```python
from build123d import *

# Parameters (mm, degrees)
F0_R     = 2.25
F0_R_2   = 6
F1_DEPTH = 2
F2_R     = 19
F2_R_2   = 6
F3_DEPTH = 4.6


with BuildPart() as f1:
    # F0 (on Top) → F1 (new body)
    with BuildSketch(Plane.XY):
        with BuildLine():
            Line((29.849623, 35), (-29.849623, 35))
            ThreePointArc((-29.849623, 35), (-32.526912, 32.526912), (-35, 29.849623))
            Line((-35, 29.849623), (-35, -29.849623))
            ThreePointArc((-35, -29.849623), (-32.526912, -32.526912), (-29.849623, -35))
            Line((-29.849623, -35), (29.849623, -35))
            ThreePointArc((29.849623, -35), (32.526912, -32.526912), (35, -29.849623))
            Line((35, -29.849623), (35, 29.849623))
            ThreePointArc((35, 29.849623), (32.526912, 32.526912), (29.849623, 35))
        make_face()
        with Locations((-27.5, -27.5)):
            Circle(F0_R, mode=Mode.SUBTRACT)
        with Locations((27.5, -27.5)):
            Circle(F0_R, mode=Mode.SUBTRACT)
        Circle(F0_R_2, mode=Mode.SUBTRACT)
        with Locations((-27.5, 27.5)):
            Circle(F0_R, mode=Mode.SUBTRACT)
        with Locations((27.5, 27.5)):
            Circle(F0_R, mode=Mode.SUBTRACT)
    extrude(amount=F1_DEPTH)

    # F2 (on face) → F3 (join)
    with BuildSketch(Plane.XY.offset(2)):
        Circle(F2_R)
        Circle(F2_R_2, mode=Mode.SUBTRACT)
    extrude(amount=-F3_DEPTH)


solid = f1.part
```
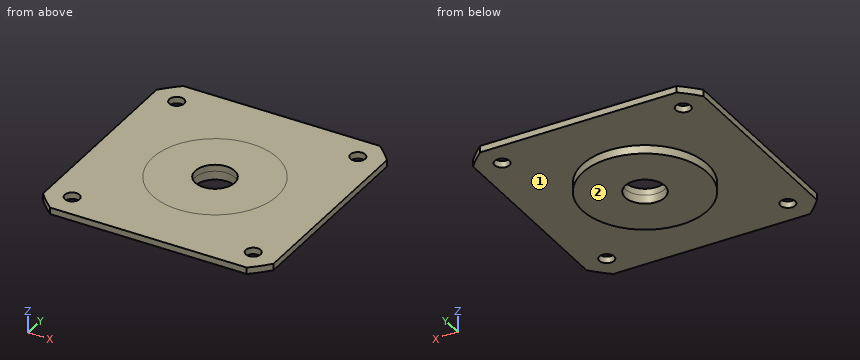
Can you work these out from the model? Positions are in its coordinate system, mm. Face numbers are marked on the shaded views. A direction names the side the tool comes from. Coordinates: 2 decimals unless noted, no trailing zeros. Write each loop counter-clockwise with the first axis right and the second up, starting at its lowest first coordinate (ties: lowest second). Pieces come first, ordered by that corner, then holes. Notation, with made-up numbers: (32.5, -38) - (54.5, -38) arc R22 ccw to (54.5, -31) - close; hole circle Ø1 at (-15.5, 31). An arc over 180 degrees is marked (long way). Return JSON: item names as keys, results as strings.
Q1. If we section it at B-B (z = 1.3): Please give me the cut outline in (x, y).
Computed values:
{"outline": "(-35, -29.85) arc R46 ccw to (-29.85, -35) - (29.85, -35) arc R46 ccw to (35, -29.85) - (35, 29.85) arc R46 ccw to (29.85, 35) - (-29.85, 35) arc R46 ccw to (-35, 29.85) - close; hole circle Ø4.5 at (-27.5, -27.5); hole circle Ø4.5 at (-27.5, 27.5); hole circle Ø12 at (0, 0); hole circle Ø4.5 at (27.5, -27.5); hole circle Ø4.5 at (27.5, 27.5)"}
Q2. On a 3-axis mill with a long thin cutter (end or side, diameter ignored), from which of +Z, -Z, +X, -X, +Y, -Y can I reach the whole of each face in a straight line? I mean the marked faces 1 and 2. Say none if no direction works.
Computed values:
{"face 1": "-Z", "face 2": "-Z, +X, -X, +Y, -Y"}
Q3. I'm going to push flat-ended pins straight in: pin 1 Ø1.5 at (x, z) = (11, -1) entering from -Y; pin 2 Ø3.5 at (x, y) = (27.5, -27.5) entering from +Z; pin 3 Ø1.5 at (y, z) = (-2, -1.5) entering from +X; pin 4 Ø5 at (x, y) = (-27.5, 27.5) entering from -Z. Where does each tip first touch, or does it pass through?
Computed values:
{"pin 1": "stops at y = -16", "pin 2": "passes through", "pin 3": "stops at x = 18.96", "pin 4": "stops at z = 0"}
Q4. Please list where these lines run through material, in increasing order: L1, parallel to Y at x = -27.5, z = 1.3; L2, parallel to Y at x = 0, z = 0.95; L3, parallel to Z at x = 30, y = 2.5. Write a range as from..to.
Computed values:
{"L1": "y = -35..-29.75, -25.25..25.25, 29.75..35", "L2": "y = -35..-6, 6..35", "L3": "z = 0..2"}
Q5. If we section it at C-C (y = 0): Please give me the cut outline in (x, z), then the cut area to 3 significant figures.
Computed values:
{"outline": "(-35, 0) - (-19, 0) - (-19, -2.6) - (-6, -2.6) - (-6, 2) - (-35, 2) - close; (6, -2.6) - (19, -2.6) - (19, 0) - (35, 0) - (35, 2) - (6, 2) - close", "area": "184 mm2"}
Q6. If we section it at A-A (x = 27.5): Please give me the cut outline in (y, z), then the cut area to 3 significant figures.
Computed values:
{"outline": "(-35, 0) - (-29.75, 0) - (-29.75, 2) - (-35, 2) - close; (-25.25, 0) - (25.25, 0) - (25.25, 2) - (-25.25, 2) - close; (29.75, 0) - (35, 0) - (35, 2) - (29.75, 2) - close", "area": "122 mm2"}
